Autodesk Inventor part; units mm, degrees
ref_plane "YZ Plane" through (0, 0, 0) normal (1, 0, 0) x (0, 1, 0)
ref_plane "XZ Plane" through (0, 0, 0) normal (0, 1, 0) x (-1, 0, 0)
ref_plane "XY Plane" through (0, 0, 0) normal (0, 0, 1) x (1, 0, 0)
sketch "Sketch1" plane through (0, 0, 0) normal (0, 0, 1) x (1, 0, 0)
  line L0 (0, 0) -> (20, 0)
  line L1 (20, 0) -> (20, 10)
  line L2 (20, 10) -> (0, 10)
  line L3 (0, 10) -> (0, 0)
  dimension "d0" = 20
  dimension "d1" = 10
extrude "Extrusion1" add sketch "Sketch1" along normal blind 10
sketch "Sketch2" plane through (0, 0, 10) normal (0, 0, 1) x (1, 0, 0)
  line L0 (0, 10) -> (0, 0) construction
  line L1 (0, 0) -> (19.8824, 10) construction
  line L2 (0, 10) -> (19.8824, 0) construction
  line L3 (6.8271, 5) -> (8.3842, 7.6969)
  line L4 (8.3842, 7.6969) -> (11.4983, 7.6969)
  line L5 (11.4983, 7.6969) -> (13.0553, 5)
  line L6 (13.0553, 5) -> (11.4983, 2.3031)
  line L7 (11.4983, 2.3031) -> (8.3842, 2.3031)
  line L8 (8.3842, 2.3031) -> (6.8271, 5)
  point P0 (9.9412, 5)
extrude "Extrusion2" add sketch "Sketch2" along normal blind 1
properties part number "Basic Sensor"
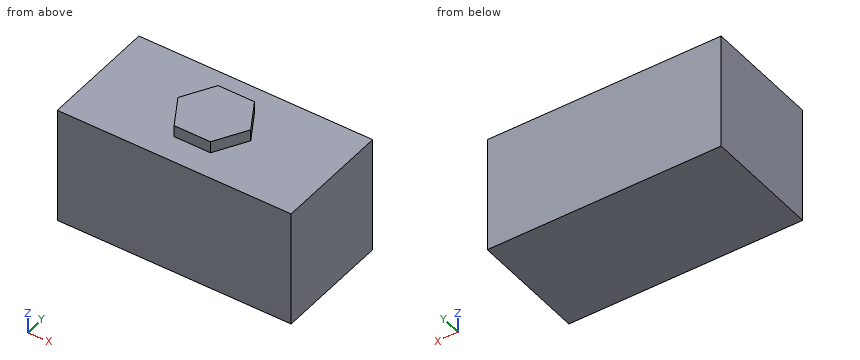
Verification items for the finished model (mm, model axes). Coordinates: 2 decimals unless noted, no trailing zeros. Order: outer loops, then holes, each group sorted by start corner. A loop starts at its lowest first (then second) coordinate and runs counter-clockwise, first axis right, second up. Notation, with made-up numbers: (-31, 29) -> (2, 29) arc R13 ccw to (2, 42) -> close; hole circle Ø7 at (-35.5, 5). An arc over 180 degrees is marked (long way). Use CSV: the item, a comma, the result in double quotes. Start each with the question number.
Q1. Section check D-D, the plane x = 5.25. Record the cut outline in (y, z).
Q2. Depth check by flat-ended pin: P1, Ø0.5, axis at x = 10.5, z = 10.5, coming from the +Y side. Enter the tip coordinate at first touch or a pass-through.
Q3. Section check B-B, the plane x = 8. Record the cut outline in (y, z).
Q4. Section check C-C, the plane y = 6.25. Record the cut outline in (x, z), and give its area (3 significant figures).
Q5. Section check A-A, the plane z = 10.25. Record the cut outline in (x, y).
Q6. Thickness scan on line 1 along Z through (x, y) = (15.75, 2.5); line 2 along Y through (x, z) = (10.75, 10.25); line 3 along X through (y, z) = (4, 10.75). Record the ranges inside material, lowest first.
Returned:
1,outline,"(0, 0) -> (10, 0) -> (10, 10) -> (0, 10) -> close"
2,P1,"stops at y = 7.7"
3,outline,"(0, 0) -> (10, 0) -> (10, 10) -> (7.03, 10) -> (7.03, 11) -> (2.97, 11) -> (2.97, 10) -> (0, 10) -> close"
4,outline,"(0, 0) -> (20, 0) -> (20, 10) -> (12.33, 10) -> (12.33, 11) -> (7.55, 11) -> (7.55, 10) -> (0, 10) -> close"
4,area,"205 mm^2"
5,outline,"(6.83, 5) -> (8.38, 2.3) -> (11.5, 2.3) -> (13.06, 5) -> (11.5, 7.7) -> (8.38, 7.7) -> close"
6,line 1,"z = 0 to 10"
6,line 2,"y = 2.3 to 7.7"
6,line 3,"x = 7.4 to 12.48"
